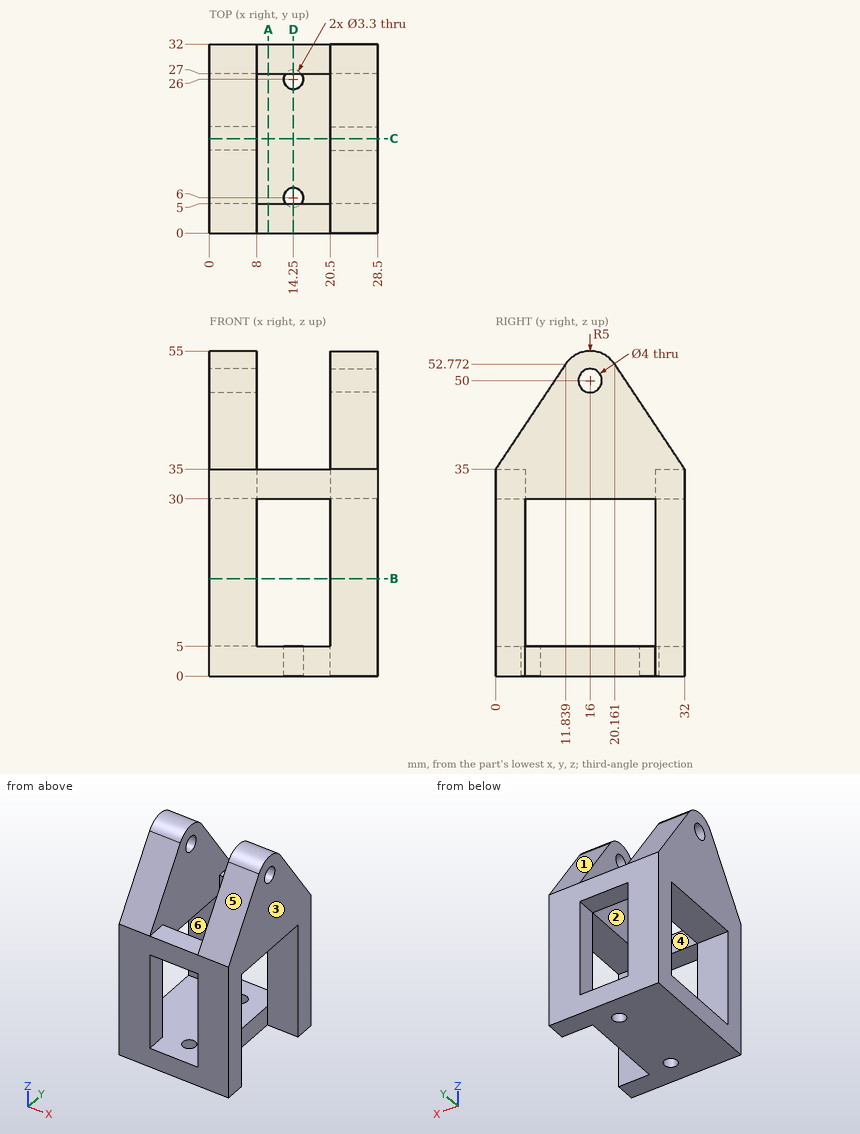
Part print with two shaded views. Sizes in mm from the minimum x, y, z corner. A direction names the side the tool comes from. Coordinates: 2 decimals unless noted, no trailing zeros. Order: outer loops, then holes, each group sorted by start corner. A loop starts at its lowest first (then second) coordinate and runs counter-clockwise, first axis right, second up.
(1) Which spindle directions (+Z, -Z, +X, -X, +Y, -Y) get a long thin tool onto all of the face, cutting with end or side? Do the marked faces 4, 5 and 6. Say none if no direction does.
Solution:
face 4: +Z
face 5: +Z, +X, -X, -Y
face 6: +X, -X
(2) Saw through at D-D, the plane x = 14.25. Write the cut outline in (y, z).
Solution:
outline: (0, 0) - (4.35, 0) - (4.35, 5) - (0, 5) - close; (0, 30) - (5, 30) - (5, 35) - (0, 35) - close; (7.65, 0) - (24.35, 0) - (24.35, 5) - (7.65, 5) - close; (27, 30) - (32, 30) - (32, 35) - (27, 35) - close; (27.65, 0) - (32, 0) - (32, 5) - (27.65, 5) - close
(3) Saw through at B-B, the plane z = 16.5. Write the cut outline in (x, y), and give its area (3 significant figures).
Solution:
outline: (0, 0) - (8, 0) - (8, 5) - (0, 5) - close; (0, 27) - (8, 27) - (8, 32) - (0, 32) - close; (20.5, 0) - (28.5, 0) - (28.5, 5) - (20.5, 5) - close; (20.5, 27) - (28.5, 27) - (28.5, 32) - (20.5, 32) - close
area: 160 mm2
(4) Saw through at C-C, the plane y = 16. Write the cut outline in (x, z).
Solution:
outline: (0, 0) - (20.5, 0) - (20.5, 5) - (0, 5) - close; (0, 30) - (8, 30) - (8, 48) - (0, 48) - close; (0, 52) - (8, 52) - (8, 55) - (0, 55) - close; (20.5, 30) - (28.5, 30) - (28.5, 48) - (20.5, 48) - close; (20.5, 52) - (28.5, 52) - (28.5, 55) - (20.5, 55) - close
(5) Drill centre lines: L1, parallel to Y at x = 14.25, z = 3.9; L2, parallel to X at y = 2, z = 18; L3, parallel to Z at x = 11.25, y = 4. Where is each one in solid material? Low to high.
Solution:
L1: y = 0 to 4.35, 7.65 to 24.35, 27.65 to 32
L2: x = 0 to 8, 20.5 to 28.5
L3: z = 0 to 5, 30 to 35
(6) Pin check, flat tips, straight feed: pin 1 Ø12 at (x, y) = (12.5, 8) entering from -Z; pin 2 Ø6 at (x, z) = (8, 39.5) entering from +Y; pin 3 Ø1.5 at (x, y) = (13.5, 3.5) entering from +Z. Stop position of each tip, or through.
Solution:
pin 1: stops at z = 0
pin 2: stops at y = 31
pin 3: stops at z = 35
(7) Mould opens along X. For the marked faces 1, 2 and 3 say: released by +X, released by -X, zero draft, split by the parting line, or undercut.
Solution:
face 1: zero draft
face 2: undercut
face 3: released by +X
(8) Saw through at A-A, the plane x = 10. Write the cut outline in (y, z), and give its area (3 significant figures).
Solution:
outline: (0, 0) - (32, 0) - (32, 5) - (0, 5) - close; (0, 30) - (5, 30) - (5, 35) - (0, 35) - close; (27, 30) - (32, 30) - (32, 35) - (27, 35) - close
area: 210 mm2
